Autodesk Inventor part; units mm, degrees
ref_plane "YZ Plane" through (0, 0, 0) normal (1, 0, 0) x (0, 1, 0)
ref_plane "XZ Plane" through (0, 0, 0) normal (0, 1, 0) x (-1, 0, 0)
ref_plane "XY Plane" through (0, 0, 0) normal (0, 0, 1) x (1, 0, 0)
sketch "Эскиз1" plane through (0, 0, 0) normal (0, 0, 1) x (1, 0, 0)
  line L0 (0, 18.7367) -> (0, -24.5413)
  arc A0 (21.6223, -7.6994) -> (21.6223, 7.6994) centre (19.45, 0) ccw
  line L1 (19.45, 0) -> (21.6223, -7.6994) construction
  line L2 (19.45, 0) -> (17.2777, 7.6994) construction
  arc A1 (-21.6223, 7.6994) -> (-19.45, -8) centre (-19.45, 0) ccw
  line L3 (-19.45, 0) -> (-19.45, 7.9959) construction
  line L4 (-19.45, 0) -> (-11.4541, 0) construction
  line L5 (-19.45, 0) -> (-19.45, -8) construction
  arc A2 (12.25, -7.6994) -> (-12.2463, -8) centre (0, -7.6994) ccw
  line L6 (-21.6223, 7.6994) -> (-3.2585, 12.8806)
  line L7 (3.2585, 12.8806) -> (21.6223, 7.6994)
  line L8 (21.6223, -7.6994) -> (12.25, -7.6994)
  line L9 (-19.45, -8) -> (-12.2463, -8)
  circle A3 centre (-19.45, 0) radius 4.5
  circle A4 centre (19.45, 0) radius 4.5
  arc A5 (3.2585, 12.8806) -> (-3.2585, 12.8806) centre (0, 1.3315) ccw
  point P0 (0, 0)
  point P1 (-27.45, 0)
  point P2 (27.45, 0)
  point P3 (0, 13.8)
  dimension "d0" = 8
  dimension "d1" = 180
  dimension "d3" = 8
  dimension "d4" = 90
  dimension "d5" = 180
  dimension "d6" = 24.5
  dimension "d7" = 54.9
  dimension "d9" = 21.8
  dimension "d10" = 9
  dimension "d11" = 9
  dimension "d12" = 12
extrude "Выдавливание1" add sketch "Эскиз1" against normal blind 13
sketch "Эскиз2" plane through (0, 0, -13) normal (0, 0, -1) x (-1, 0, 0)
  circle A0 centre (0, -8) radius 15.475
  point P0 (0, 0)
  point P1 (12.2463, -8)
  dimension "d15" = 30.95
extrude "Выдавливание2" cut sketch "Эскиз2" against normal blind 6.2
fillet "Сопряжение1" radius 0.5 1 edges at (-0.1503, 7.4743, -6.8)
chamfer "Фаска1" distance 0.5 angle 45 1 edges at (-0.1503, 7.4743, -13) measured on face at (-11.2492, 8.421, -13)
chamfer "Фаска2" distance 0.5 angle 45 1 edges at (-0.1503, 4.5497, -6.8) measured on face at (13.8976, -6.5154, -6.8)
properties part number "50073 Полуфланец"
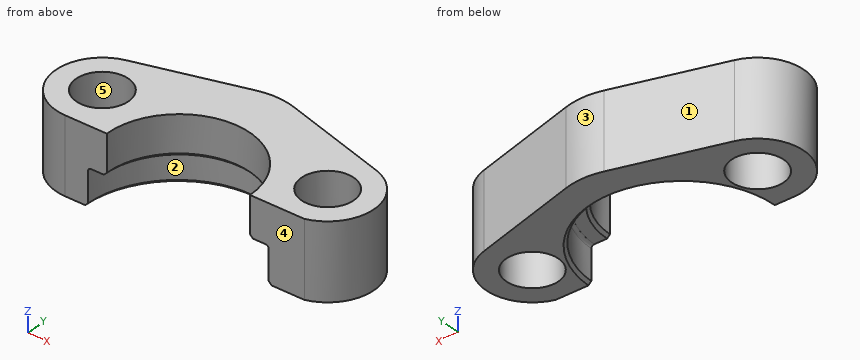
Geometry: final body of the model. Coordinates: model frame, mm. Face numbers are marked on the shaded views. A direction names the side the tool comes from. Coordinates: 2 decimals unless noted, no trailing zeros. Loops run counter-clockwise (first coordinate to the right, second up) from the corner with the lowest first, then second, coordinate; pieces in that order, holes last. Notation, with made-up numbers: (39.25, 45) - (94.25, 45) arc R18 ccw to (94.25, 70) - close; hole circle Ø3 at (46.5, 2.5). An arc over 180 degrees is marked (long way). Put each result on its own line as item: value. Start each with the question number.
Q1. Line query: line 1 (X direction, y = 0.5, z = -11.75); line 2 (Z direction, x = 13.5, y = -4); line 3 (X direction, y = 2.75, z = -9.75). Output: solid intervals per line, ascending.
Q2. Cut plane A-A, the plane z = -5.5. Return loops of the section in (x, y).
Q3. Pin query (flat end, axial travel): pin 1 Ø1 at (x, z) = (5.5, -5.5) entering from -Y; pin 2 Ø2 at (x, z) = (21, -7.5) entering from -Y; pin 3 Ø6 at (x, z) = (14, -2.5) entering from +Y. Return the tip coordinate at first contact, or that it passes through.
Q4. Cut plane B-B, the plane x = 19.45. Return loops of the section in (y, z).
Q5. Cut plane C-C, the plane y = -1.75. Give the number of separate pieces and of enclosed holes in the cut face, and give its area (3 significant figures).
Q6. Set-up query: the marked faces 1 and 2. Return all of +Z, -Z, +X, -X, +Y, -Y with unobstructed straight access to the full face (end or side cutting, diameter ignored); none if empty.
Q7. Pull-direction query (X, two-part tool) for the marked faces 3, 4 and 5; classes: released by +X, released by -X, zero draft, split by the parting line, or undercut.
Filled sheet:
1. line 1: -27.43 to -23.92, -14.98 to -12.93, 12.93 to 14.98, 23.92 to 27.43
1. line 2: -6.8 to 0
1. line 3: -26.96 to -23.01, -15.89 to -11.13, 11.13 to 15.89, 23.01 to 26.96
2. outline: (-21.62, 7.7) arc R8 ccw to (-19.45, -8) - (-12.25, -8) arc R12.25 cw (long way) to (12.25, -7.7) - (21.62, -7.7) arc R8 ccw to (21.62, 7.7) - (3.26, 12.88) arc R12 ccw to (-3.26, 12.88) - close; hole circle Ø9 at (-19.45, 0); hole circle Ø9 at (19.45, 0)
3. pin 1: y = 2.98
3. pin 2: y = -7.7
3. pin 3: y = 10.7
4. outline: (-7.7, -13) - (-4.5, -13) - (-4.5, 0) - (-7.7, 0) - close; (4.5, -13) - (8.31, -13) - (8.31, 0) - (4.5, 0) - close
5. separate pieces: 4
5. enclosed holes: 0
5. area: 171 mm²
6. face 1: +Z, -Z, -X, +Y
6. face 2: -Z, -Y
7. face 3: split by the parting line
7. face 4: zero draft
7. face 5: undercut
